```python
from build123d import *

# Parameters (mm, degrees)
F0_W     = 90
F0_H     = 154
F0_W_2   = 85
F0_H_2   = 150
F0_W_3   = 80
F0_H_3   = 146
F1_DEPTH = 3
F2_DEPTH = 50
F3_DEPTH = 52
F4_R     = 5
F5_DEPTH = 5


with BuildPart() as f1:
    # F0 (on Top) → F1 (new body)
    with BuildSketch(Plane.XY):
        Rectangle(F0_W, F0_H)
        Rectangle(F0_W_2, F0_H_2, mode=Mode.SUBTRACT)
        Rectangle(F0_W_2, F0_H_2)
        Rectangle(F0_W_3, F0_H_3, mode=Mode.SUBTRACT)
        Rectangle(F0_W_3, F0_H_3)
    extrude(amount=F1_DEPTH)

    # F0 (on Top) → F2 (join)
    with BuildSketch(Plane.XY):
        Rectangle(F0_W, F0_H)
        Rectangle(F0_W_2, F0_H_2, mode=Mode.SUBTRACT)
        Rectangle(F0_W_2, F0_H_2)
        Rectangle(F0_W_3, F0_H_3, mode=Mode.SUBTRACT)
    extrude(amount=-F2_DEPTH)

    # F0 (on Top) → F3 (join)
    with BuildSketch(Plane.XY):
        Rectangle(F0_W, F0_H)
        Rectangle(F0_W_2, F0_H_2, mode=Mode.SUBTRACT)
    extrude(amount=-F3_DEPTH)

    # F4 (on face) → F5 (cut)
    with BuildSketch(Plane(origin=(0, 77, 0), x_dir=(-1, 0, 0), z_dir=(0, 1, 0))):
        with Locations((0, -7)):
            Circle(F4_R)
    extrude(amount=-F5_DEPTH, mode=Mode.SUBTRACT)


solid = f1.part
```
CAD build for the part. Positions are in the model's coordinates, mm. A direction names the side the tool comes from. Coordinates: 2 decimals unless noted, no trailing zeros. Order: outer loops, then holes, each group sorted by start corner. A loop starts at its lowest first (then second) coordinate and runs counter-clockwise, first axis right, second up. Notation, with made-up numbers: (33.25, 23) -> (90.25, 23) arc R25 cw to (90.25, 61) -> close; hole circle Ø11 at (-36, 41). An arc over 180 degrees is marked (long way). Use one line per item in the form item = value. Start each with the question number.
1) Tool access for faces 4 (the cylindrical face through (-3, 75, -3)), 5 (the flat face through (-1, 1, 3)), 6 (the flat face through (40, -1, -25)): list every direction of +Z, -Z, +X, -X, +Y, -Y with a clear straight run to the whole face (end or side of a thin tool).
2) Pull direction X, two halves, no side cores. Call faces 1 (the flat face through (-41, 0, -50)), 2 (the flat face through (-45, -1, -24)), 3 (the flat face through (43, 0, -52)): +X half, -X half, draft (parallel to the pull), parting line (faces both ways), or undercut.
3) Drill centre lines: L1, parallel to Z at x = 0, y = 74.75; L2, parallel to Y at x = -5, z = -35; L3, parallel to X at y = 38, z = -39.5. Where is each one in solid material? Low to high. Write a range as [from, to].
4) Band-saw the part on D-D on z = -7. Give the cut face in (x, y), then the cut area to 3 significant figures.
5) Drop flat-ended pins along their axis: pin 1 (8 mm diameter, centred on x = 0, z = -7, fed in from +Y); pin 2 (1 mm diameter, centred on x = -33.5, y = 40, fed in from -Z). Give the stop position or say it passes through.
6) Band-saw the part on A-A on x = 0. Give the cut face in (y, z).
7) Band-saw the part on C-C on z = -21. Give the cut face in (x, y).
8) Band-saw the part on B-B on y = 1. Give the cut face in (x, z).
Entries:
q1.face_4 = +Y
q1.face_5 = +Z, +X, -X, +Y, -Y
q1.face_6 = -Z
q2.face_1 = undercut
q2.face_2 = -X half
q2.face_3 = draft
q3.L1 = [-50, -12], [-2, 3]
q3.L2 = [-77, -73], [73, 77]
q3.L3 = [-45, -40], [40, 45]
q4.outline = (-45, -77) -> (45, -77) -> (45, 77) -> (5, 77) -> (5, 73) -> (40, 73) -> (40, -73) -> (-40, -73) -> (-40, 73) -> (-5, 73) -> (-5, 77) -> (-45, 77) -> close
q4.area = 2,140 mm2
q5.pin_1 = -73
q5.pin_2 = 0
q6.outline = (-77, -52) -> (-75, -52) -> (-75, -50) -> (-73, -50) -> (-73, 0) -> (73, 0) -> (73, -2) -> (77, -2) -> (77, 3) -> (-77, 3) -> close; (73, -50) -> (75, -50) -> (75, -52) -> (77, -52) -> (77, -12) -> (73, -12) -> close
q7.outline = (-45, -77) -> (45, -77) -> (45, 77) -> (-45, 77) -> close; hole (-40, -73) -> (40, -73) -> (40, 73) -> (-40, 73) -> close
q8.outline = (-45, -52) -> (-42.5, -52) -> (-42.5, -50) -> (-40, -50) -> (-40, 0) -> (40, 0) -> (40, -50) -> (42.5, -50) -> (42.5, -52) -> (45, -52) -> (45, 3) -> (-45, 3) -> close
